Design review of the part built by this model. Coordinates are the model's own, in mm. A direction names the side the tool comes from. Round coordinates to 2 decimals unless told otherwise and drop trailing zeros. Order: outer loops, then holes, each group sorted by start corner. A loop starts at its lowest first (then second) coordinate and runs counter-clockwise, first axis right, second up. Notation, with made-up numbers: M -29,5.5 L 9,5.5 A10 ccw 9,13.5 Z; hole C 18.25,43 d4. An arc over 180 degrees is marked long. Use a Markdown table: item, result. Add a question column.
(1) The part is to be moulded in two halves that separate along Y. For faces 1 (the face through (-1, -38.5, 27)), 2 (the face through (75, -1, 28)), 3 (the face through (66.6, -1.8, 5.1)), 4 (the face through (-1, 38.5, 27)), say which applies: released by +Y, released by -Y, zero draft, split by the parting line, or undercut.
(2) To check wall thickness, follow probe 1 along Z at (x, y) = (-65, 4.5); probe 2 along Y at (x, z) = (69, 26); probe 3 along X at (y, z) = (0.5, 7). State the ranges of each line that lie inside material, in increasing order. Write a range as from..to.
(3) For pin 1 (4 mm diameter, centred on y = -21.5, z = 16.5, fed in from +X); pin 2 (0.6 mm diameter, centred on y = -3.5, z = 16.5, fed in from -X), all flat-tipped, find the tip position at first contact; note any pin that passes through.
(4) Take a section at A-A (y = 0). Count the separate pieces of the cut face and the enclosed holes in it, then the cut area to 3 significant figures.
(5) Take a section at C-C (z = 24). Write out the cut boundary in (x, y).
(6) Take a section at D-D (y = 13.5). Write out the cut boundary in (x, z).
(7) Take a section at B-B (x = 69). Write out the cut boundary in (y, z), then the cut area to 3 significant figures.
(8) Machinability: for faces 5 (the face through (73, -1, 10)), 6 (the face through (0.572, -0.539, 25.994)), 7 (the face through (-58.804, -0.539, 11.711)), which of the approach directions +Z, -Z, +X, -X, +Y, -Y give a long, thin tool a straight path to every point of the face, cutting with its end or side? Answer none if there is none.
```python
from build123d import *

# Parameters (mm, degrees)
BOSS_EXTRUDE1_DEPTH      = 38.5
BOSS_EXTRUDE1_DEPTH_BACK = 38.5
SKETCH5_R                = 3
CUT_EXTRUDE1_DEPTH       = 91.352089074


with BuildPart() as part:
    # Sketch1 → Boss-Extrude1 (new, two sides: drawn at the far end of the back side and taken through both)
    with BuildSketch(Plane(origin=(0, 0, 0), x_dir=(1, 0, 0), z_dir=(0, 1, 0)).offset(-BOSS_EXTRUDE1_DEPTH_BACK)):
        with BuildLine():
            Line((-26, 0), (-75, 0))
            Line((-75, 0), (-75, -10))
            Line((-75, -10), (-63, -10))
            ThreePointArc((-63, -10), (-58.757359313, -11.757359313), (-57, -16))
            Line((-57, -16), (-57, -16.5))
            ThreePointArc((-57, -16.5), (-58.757359313, -20.742640687), (-63, -22.5))
            Line((-63, -22.5), (-75, -22.5))
            Line((-75, -22.5), (-75, -32.5))
            Line((-75, -32.5), (75, -32.5))
            Line((75, -32.5), (75, -22.5))
            Line((75, -22.5), (63, -22.5))
            ThreePointArc((63, -22.5), (58.757359313, -20.742640687), (57, -16.5))
            Line((57, -16.5), (57, -16))
            ThreePointArc((57, -16), (58.757359313, -11.757359313), (63, -10))
            Line((63, -10), (75, -10))
            Line((75, -10), (75, 0))
            Line((75, 0), (26, 0))
            ThreePointArc((26, 0), (0, -26), (-26, 0))
        make_face()
    extrude(amount=BOSS_EXTRUDE1_DEPTH + BOSS_EXTRUDE1_DEPTH_BACK)

    # Sketch5 → Cut-Extrude1 (cut, through all)
    with BuildSketch(Plane.XY.offset(32.5)):
        with Locations((-69, 0)):
            Circle(SKETCH5_R)
        with Locations((69, 0)):
            Circle(SKETCH5_R)
    extrude(amount=-CUT_EXTRUDE1_DEPTH, mode=Mode.SUBTRACT)


solid = part.part
```
Verdict:
| question | item | result |
|---|---|---|
| 1 | face 1 | released by -Y |
| 1 | face 2 | zero draft |
| 1 | face 3 | undercut |
| 1 | face 4 | released by +Y |
| 2 | probe 1 | z = 0..10, 22.5..32.5 |
| 2 | probe 2 | y = -38.5..-3, 3..38.5 |
| 2 | probe 3 | x = -75..-71.96, -66.04..-25.04, 25.04..66.04, 71.96..75 |
| 3 | pin 1 | stops at x = 57.34 |
| 3 | pin 2 | stops at x = -57.01 |
| 4 | separate pieces | 5 |
| 4 | enclosed holes | 0 |
| 4 | area | 3,150 mm^2 |
| 5 | outline | M -75,-38.5 L -10,-38.5 L -10,38.5 L -75,38.5 Z; M 10,-38.5 L 75,-38.5 L 75,38.5 L 10,38.5 Z; hole C -69,0 d6; hole C 69,0 d6 |
| 6 | outline | M -75,0 L -26,0 A26 cw 26,0 L 75,0 L 75,10 L 63,10 A6 cw 57,16 L 57,16.5 A6 cw 63,22.5 L 75,22.5 L 75,32.5 L -75,32.5 L -75,22.5 L -63,22.5 A6 cw -57,16.5 L -57,16 A6 cw -63,10 L -75,10 Z |
| 7 | outline | M -38.5,0 L -3,0 L -3,10 L -38.5,10 Z; M -38.5,22.5 L -3,22.5 L -3,32.5 L -38.5,32.5 Z; M 3,0 L 38.5,0 L 38.5,10 L 3,10 Z; M 3,22.5 L 38.5,22.5 L 38.5,32.5 L 3,32.5 Z |
| 7 | area | 1,420 mm^2 |
| 8 | face 5 | +X, +Y, -Y |
| 8 | face 6 | -Z, +Y, -Y |
| 8 | face 7 | -X, +Y, -Y |
